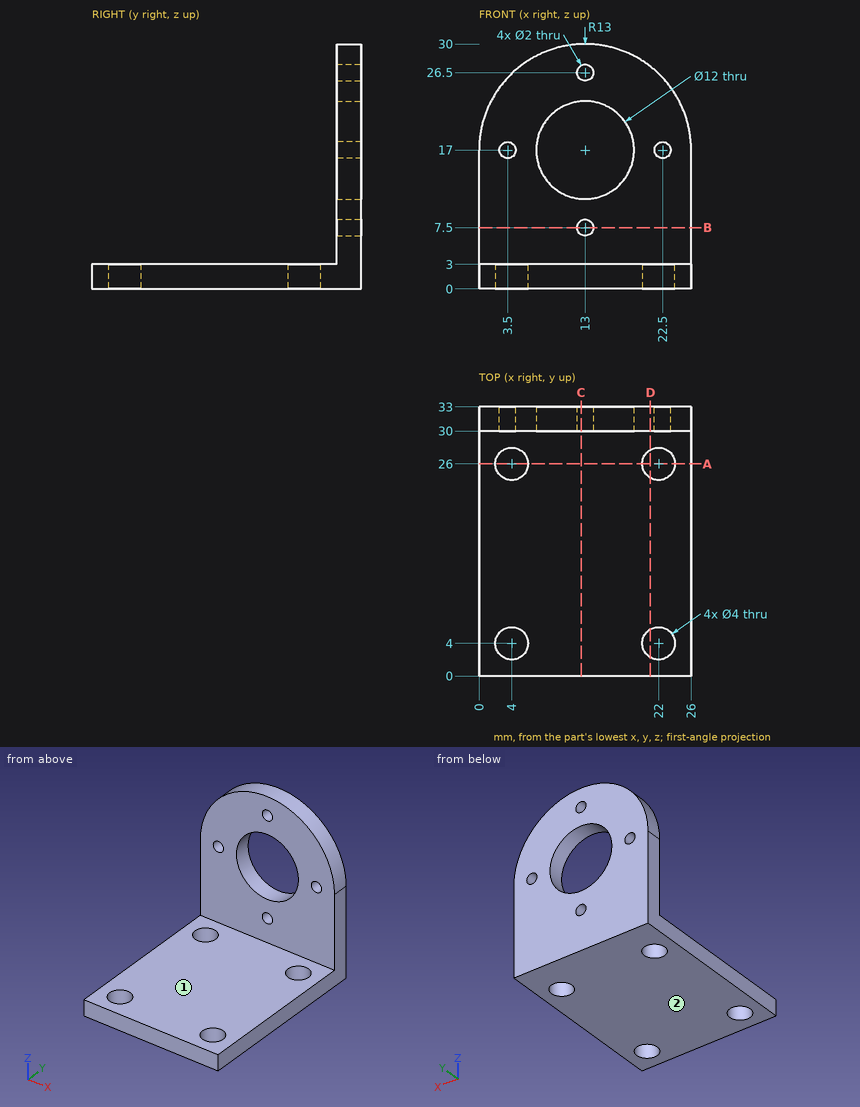
The figure shows three views and two pictorial views of one solid part (mm, origin at its lowest corner). Answer the questions. A direction names the side the tool comes from. Coordinates: 2 decimals unless noted, no trailing zeros. Order: outer loops, then holes, each group sorted by start corner. A loop starts at its lowest first (then second) coordinate and runs counter-clockwise, first axis right, second up. Notation, with made-up numbers: (-36.75, 38.25) - (-19.75, 38.25) arc R8 cw to (-19.75, 53.25) - close; hole circle Ø8 at (73.25, 0). An arc over 180 degrees is marked (long way). Answer as a JSON object with one key per item and string values.
1. A tool of negligible diameter and unlimited length cuts with its end or side. For the marked faces 1 and 2, from which of +Z, -Z, +X, -X, +Y, -Y can it reach the whole face along a straight path? Write none if from no direction.
Output values:
{"face 1": "+Z, +X, -X, -Y", "face 2": "-Z, +X, -X, +Y, -Y"}
2. Consider line 1 (Z direction, x = 13, y = 30.8); line 2 (X direction, y = 26, z = 1); line 3 (Y direction, x = 22, z = 0.7). Determine where each line is inside the solid, lowest interval first.
Output values:
{"line 1": "z = 0 to 6.5, 8.5 to 11, 23 to 25.5, 27.5 to 30", "line 2": "x = 0 to 2, 6 to 20, 24 to 26", "line 3": "y = 0 to 2, 6 to 24, 28 to 33"}
3. Find section A-A on y = 26. Determine the outline of the cut face in (x, z), plus the area to 3 significant figures.
Output values:
{"outline": "(0, 0) - (2, 0) - (2, 3) - (0, 3) - close; (6, 0) - (20, 0) - (20, 3) - (6, 3) - close; (24, 0) - (26, 0) - (26, 3) - (24, 3) - close", "area": "54.0 mm²"}
4. Find section D-D on x = 21. Determine the outline of the cut face in (y, z), plus the area to 3 significant figures.
Output values:
{"outline": "(0, 0) - (2.27, 0) - (2.27, 3) - (0, 3) - close; (5.73, 0) - (24.27, 0) - (24.27, 3) - (5.73, 3) - close; (27.73, 0) - (33, 0) - (33, 27.25) - (30, 27.25) - (30, 3) - (27.73, 3) - close", "area": "151 mm²"}
5. Find section B-B on z = 7.5. Determine the outline of the cut face in (x, y), plus the area to 3 significant figures.
Output values:
{"outline": "(0, 30) - (12, 30) - (12, 33) - (0, 33) - close; (14, 30) - (26, 30) - (26, 33) - (14, 33) - close", "area": "72.0 mm²"}
6. Find section C-C on x = 12.5. Determine the outline of the cut face in (y, z), plus the area to 3 significant figures.
Output values:
{"outline": "(0, 0) - (33, 0) - (33, 6.63) - (30, 6.63) - (30, 3) - (0, 3) - close; (30, 8.37) - (33, 8.37) - (33, 11.02) - (30, 11.02) - close; (30, 22.98) - (33, 22.98) - (33, 25.63) - (30, 25.63) - close; (30, 27.37) - (33, 27.37) - (33, 29.99) - (30, 29.99) - close", "area": "134 mm²"}
7. Each of these flat-tipped pins is pushed along its axis until it touches: P1, Ø3, axis at x = 3.5, z = 17, coming from the -Y side; P2, Ø1, axis at x = 8.5, y = 8.5, coming from the +Z side. Where does it stop, or does it pass through?
Output values:
{"P1": "stops at y = 30", "P2": "stops at z = 3"}
